CAD build for the part. Positions are in the model's coordinates, mm. A direction names the side the tool comes from. Round coordinates to 2 decimals unless told otherwise and drop trailing zeros. Loops run counter-clockwise (first coordinate to the right, second up) from the corner with the lowest first, then second, coordinate; pieces in that order, holes last.
from build123d import *

# Parameters (mm, degrees)
SKETCH1_R           = 50
SKETCH1_R_2         = 40
SKETCH1_R_3         = 10
BOSS_EXTRUDE1_DEPTH = 80
SKETCH6_W           = 60
SKETCH6_H           = 50


with BuildPart() as part:
    # Sketch1 → Boss-Extrude1 (new body)
    # profile 1 of 4: a face of its own
    with BuildSketch(Plane.XY):
        Circle(SKETCH1_R)
        Circle(SKETCH1_R_2, mode=Mode.SUBTRACT)
    # profile 2 of 4: a face of its own
    with BuildSketch(Plane.XY):
        with BuildLine():
            ThreePointArc((20, 70), (0, 90), (-20, 70))
            Line((-20, 70), (-20, 45.82575695))
            ThreePointArc((-20, 45.82575695), (0, 50), (20, 45.82575695))
            Line((20, 45.82575695), (20, 70))
        make_face()
        with Locations((0, 70)):
            Circle(SKETCH1_R_3, mode=Mode.SUBTRACT)
    # profile 3 of 4: a face of its own
    with BuildSketch(Plane.XY):
        with BuildLine():
            ThreePointArc((-29.686269666, -40.23338655), (-43.301270189, -25), (-49.686269666, -5.592370399))
            Line((-49.686269666, -5.592370399), (-70.621778265, -17.679491924))
            ThreePointArc((-70.621778265, -17.679491924), (-77.942286341, -45), (-50.621778265, -52.320508076))
            Line((-50.621778265, -52.320508076), (-29.686269666, -40.23338655))
        make_face()
        with Locations((-60.621778265, -35)):
            Circle(SKETCH1_R_3, mode=Mode.SUBTRACT)
    # profile 4 of 4: a face of its own
    with BuildSketch(Plane.XY):
        with BuildLine():
            Line((70.621778265, -17.679491924), (49.686269666, -5.592370399))
            ThreePointArc((49.686269666, -5.592370399), (43.301270189, -25), (29.686269666, -40.23338655))
            Line((29.686269666, -40.23338655), (50.621778265, -52.320508076))
            ThreePointArc((50.621778265, -52.320508076), (77.942286341, -45), (70.621778265, -17.679491924))
        make_face()
        with Locations((60.621778265, -35)):
            Circle(SKETCH1_R_3, mode=Mode.SUBTRACT)
    extrude(amount=BOSS_EXTRUDE1_DEPTH)

    # Sketch6 → Cut-Revolve1 (revolve, cut)
    with BuildSketch(Plane(origin=(0, 0, 0), x_dir=(-0.8660254037844385, -0.5000000000000004, 0), z_dir=(0.5000000000000003, -0.8660254037844384, 0)), mode=Mode.PRIVATE) as cut_revolve1_sk:
        with Locations((80, -40)):
            Rectangle(SKETCH6_W, SKETCH6_H)
    revolve(cut_revolve1_sk.sketch.rotate(Axis((0, 0, 80), (0, 0, -1)), 23.578178478), axis=Axis((0, 0, 80), (0, 0, -1)), mode=Mode.SUBTRACT)


solid = part.part
Item 1: Flat gauge pins, fed straight in: P1, Ø18, axis at x = 0, y = 70, coming from the -Z side; P2, Ø6, axis at x = -28, z = 38.5, coming from the +Y side; P3, Ø4.5, axis at y = 52, z = 69, coming from the -X side; P4, Ø15, axis at x = -62, y = -28, coming from the +Z side. Where does each tip first touch, or does it go through?
Verdict:
P1: passes through
P2: stops at y = 43.3
P3: stops at x = -20
P4: stops at z = 80
Item 2: Cut at D-D (x = -38). List the corners of the cut face in (y, z), plus the area to 3 significant figures.
Verdict:
outline: (-45.03, 0) - (-12.49, 0) - (-12.49, 80) - (-45.03, 80) - (-45.03, 65) - (-32.5, 65) - (-32.5, 15) - (-45.03, 15) - close; (12.49, 0) - (32.5, 0) - (32.5, 80) - (12.49, 80) - close
area: 3,580 mm2
Item 3: Cut at C-C (y = -35). State how many separate pieces and enclosed holes the cut face has, plus the area to 3 significant figures.
Verdict:
separate pieces: 6
enclosed holes: 0
area: 4,110 mm2
Item 4: Mould opens along X. For faces 1 (the flat face through (49, -36, 65)), 2 (the flat face through (-60.007, -11.551, 7.395)), 3 (the flat face through (-40.3, -46.36, 7.4)), 4 (the flat face through (20, 58, 7)) say: released by +X, released by -X, zero draft, split by the parting line, or undercut.
Verdict:
face 1: zero draft
face 2: released by -X
face 3: undercut
face 4: released by +X
Item 5: Cut at A-A (y = 0). List the corners of the cut face in (x, z).
Verdict:
outline: (-50, 0) - (-40, 0) - (-40, 80) - (-50, 80) - close; (40, 0) - (50, 0) - (50, 80) - (40, 80) - close
Item 6: Cut at B-B (x = 0). List the corners of the cut face in (y, z), plus the area to 3 significant figures.
Verdict:
outline: (-50, 0) - (-40, 0) - (-40, 80) - (-50, 80) - close; (40, 0) - (60, 0) - (60, 15) - (50, 15) - (50, 65) - (60, 65) - (60, 80) - (40, 80) - close; (80, 0) - (90, 0) - (90, 15) - (80, 15) - close; (80, 65) - (90, 65) - (90, 80) - (80, 80) - close
area: 2,200 mm2
Item 7: Wall check: L1, parallel to Y at x = 0, z = 4; L2, parallel to Z at x = 2, y = 83; L3, parallel to Y at x = 4, z = 14. Give the ranges that are in metal, low to high.
Verdict:
L1: y = -50 to -40, 40 to 60, 80 to 90
L2: z = 0 to 15, 65 to 80
L3: y = -49.84 to -39.8, 39.8 to 60.83, 79.17 to 89.6
Item 8: 3-axis set-ups, long thin cutter, end or side, ignore diameter. For faces 5 (the flat face through (-20, 58, 7)), 6 (the flat face through (40.007, -46.192, 7.395)), 7 (the cylindrical face through (5.38, 78.43, 7.4)), 8 (the flat face through (-50, -35, 65)), 9 (the flat face through (-36, 18, 80)): which of +Z, -Z, +X, -X, +Y, -Y reach the whole face in a straight line?
Verdict:
face 5: +Z, -Z, -X, +Y
face 6: +Z, -Z, -Y
face 7: +Z, -Z
face 8: -X, -Y
face 9: +Z, +X, -X, +Y, -Y
